Job drawing, mm, ordinate dimensions from the low corner. One solid piece. Give positions to 0.01 mm unless a question says otherwise; leave off trailing zeros. Order: outer loops, then holes, each group sorted by start corner. A loop starts at its lowest first (then second) coordinate and runs counter-clockwise, first axis right, second up. Notation, with made-up numbers: (0, 33.5) - (53, 33.5) arc R6 ccw to (53, 43.5) - close; hole circle Ø7 at (63, 0). An arc over 180 degrees is marked (long way). One line per item, written item: value.
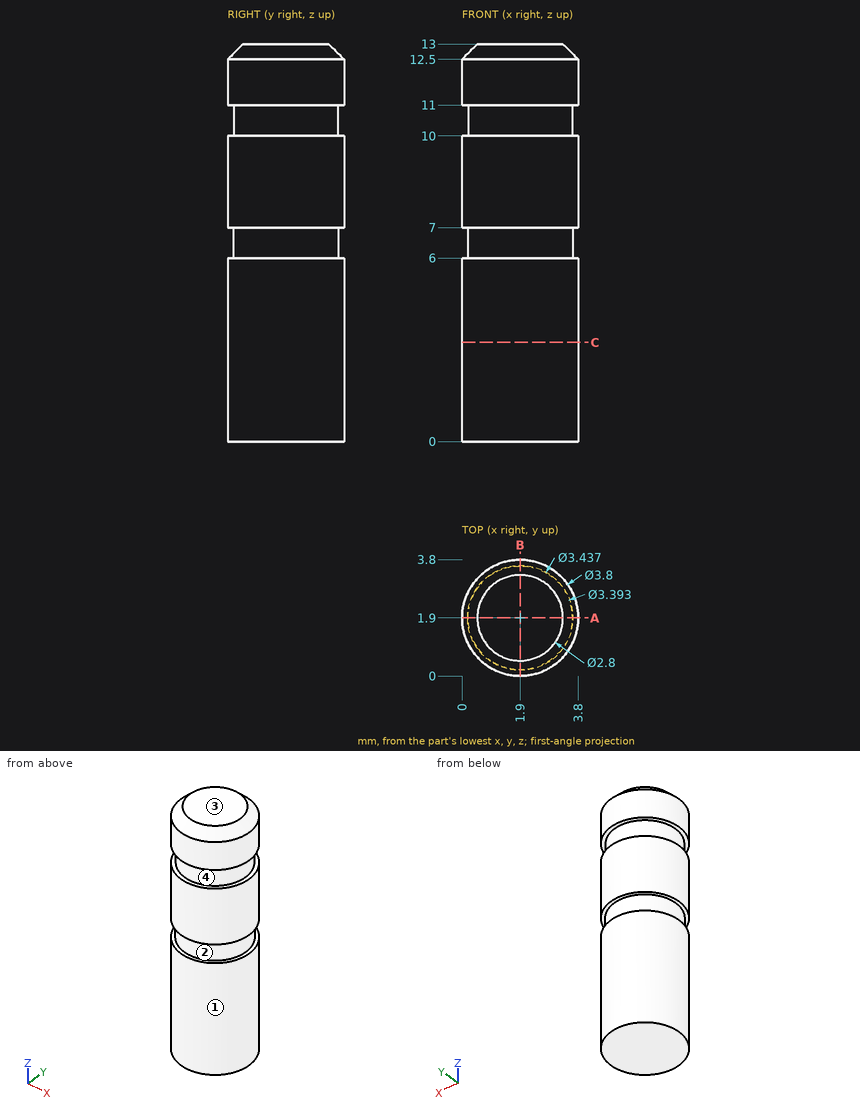
1) Slice it at C-C on z = 3.25. Write the cut outline in (x, y).
Answer:
outline: circle Ø3.8 at (1.9, 1.9)
2) Two-plate mould, pull along Z, no slides. Class the marked faces 1, 2, 3 and 4: pulls with the +Z half, pulls with the -Z half, needs draft (parallel to the pull), parting line crosses it, or undercut.
Answer:
face 1: needs draft
face 2: undercut
face 3: pulls with the +Z half
face 4: undercut
3) Wall check: line 1 along Z through (x, y) = (1.15, 3.6); line 2 along X through (y, z) = (3.2, 2.5) (1 decimal); line 3 along X through (y, z) = (2.55, 11.75) (1 decimal). Give the ranges that are in metal, low to high. Write a range as [from, to].
Answer:
line 1: z = [0, 6], [7, 10], [11, 12.54]
line 2: x = [0.5, 3.3]
line 3: x = [0.1, 3.7]
4) Slice it at A-A on y = 1.9. Write the cut outline in (x, z).
Answer:
outline: (0, 0) - (3.8, 0) - (3.8, 6) - (3.62, 6) - (3.62, 7) - (3.8, 7) - (3.8, 10) - (3.6, 10) - (3.6, 11) - (3.8, 11) - (3.8, 12.5) - (3.3, 13) - (0.5, 13) - (0, 12.5) - (0, 11) - (0.2, 11) - (0.2, 10) - (0, 10) - (0, 7) - (0.18, 7) - (0.18, 6) - (0, 6) - close
